Work out the finished part from the listing and answer in its coordinate system (mm). A direction names the side the tool comes from. Round coordinates to 2 decimals unless told otherwise and drop trailing zeros. Write each loop counter-clockwise with the first axis right and the second up, starting at its lowest first coordinate (ties: lowest second). Pieces come first, ordered by that corner, then holes. Notation, with made-up numbers: M 73.25,88 L 87.25,88 A25 cw 87.25,118 Z; hole C 85.5,22 d10. An arc over 180 degrees is marked long. Answer in a Markdown table with one row per item.
```python
from build123d import *

# Parameters (mm, degrees)
F1_DEPTH = 10
F2_R     = 7
F3_SIZE  = 2.99999


# Not quite as in the source:
# - a fillet or chamfer is up to 0.001 mm smaller than in the source, because OpenCascade refuses the exact size


with BuildPart() as f1:
    # F0 (on Top) → F1 (new body)
    with BuildSketch(Plane.XY):
        with BuildLine():
            Line((-20, 0), (0, 0))
            Line((0, 0), (0, -20))
            ThreePointArc((0, -20), (5.4462447196, 5.4462447196), (-20, 0))
        make_face()
    extrude(amount=F1_DEPTH)

    # F2
    f2_edges = [f1.edges().sort_by_distance(p)[0] for p in [
        (5.446245, 5.446245, 10),
    ]]
    fillet(f2_edges, radius=F2_R)

    # F3 (size 3 in the source; OpenCascade refuses exactly that, so slightly less here)
    f3_edges = [f1.edges().sort_by_distance(p)[0] for p in [
        (5.446245, 5.446245, 0),
    ]]
    chamfer(f3_edges, length=F3_SIZE)


solid = f1.part
```
1. The part is cut by section B-B (z = 4). Determine the outline of the cut face in (x, y), plus the area to 3 significant figures.
Calculated:
| item | result |
|---|---|
| outline | M -19.92,0 L 0,0 L 0,-19.92 A15.43 ccw long Z |
| area | 364 mm² |
2. Consider line 1 along Z through (x, y) = (4.25, -16); line 2 along Y through (x, z) = (-1.5, 5.5); line 3 along Z through (x, y) = (-15.5, 2.5). Determine where each line is inside the solid, lowest interval first. Write a range as from..to.
Calculated:
| item | result |
|---|---|
| line 1 | z = 1.83..6.88 |
| line 2 | y = 0..8.98 |
| line 3 | z = 0.3..8.52 |
3. A tool of negligible diameter and unlimited length cuts with its end or side. For faces 1 (the flat face through (0, -10, 5)), 2 (the flat face through (0.5, -1.7, 10)), from which of +Z, -Z, +X, -X, +Y, -Y can it reach the whole face along a straight path? Write none if from no direction.
Calculated:
| item | result |
|---|---|
| face 1 | +Z, -Z, -X, -Y |
| face 2 | +Z, +X, -X, +Y, -Y |
4. Given pin 1 (2 mm diameter, centred on y = 3, z = 5.5, fed in from +X); pin 2 (3 mm diameter, centred on x = -11, z = 8.5, fed in from +Y), each flat-ended and moving along its own axis, determine where each tip first touches the part or whether it passes through.
Calculated:
| item | result |
|---|---|
| pin 1 | stops at x = 7.63 |
| pin 2 | stops at y = 7.77 |
5. The part is cut by section A-A (z = 8). Determine the outline of the cut face in (x, y).
Calculated:
| item | result |
|---|---|
| outline | M -17.73,0 L 0,0 L 0,-17.73 A13.4 ccw long Z |
